Model file for the job. Use its own axes, mm. A direction names the side the tool comes from. Coordinates: 2 decimals unless noted, no trailing zeros. Order: outer loops, then holes, each group sorted by start corner. A loop starts at its lowest first (then second) coordinate and runs counter-clockwise, first axis right, second up.
from build123d import *

# Parameters (mm, degrees)
SKETCH2_W               = 180
SKETCH2_H               = 9
BOSS_EXTRUDE1_DEPTH     = 14.8
SKETCH7_W               = 180
SKETCH7_H               = 4.5
CUT_EXTRUDE1_DEPTH      = 92.319713096
SKETCH8_W               = 90
SKETCH8_H               = 4.5
BOSS_EXTRUDE2_DEPTH     = 7
SKETCH10_R              = 1.5
CUT_EXTRUDE2_DEPTH      = 8
BOSS_EXTRUDE3_DEPTH     = 14.8
CUT_EXTRUDE3_DEPTH      = 178.187961437
CUT_EXTRUDE3_DEPTH_BACK = 178.187961437
SKETCH12_R              = 2
CUT_EXTRUDE4_DEPTH      = 112.397156258
CUT_EXTRUDE4_DEPTH_BACK = 112.397156258
SKETCH13_W              = 26.348017916
SKETCH13_H              = 14.929639375
FILLET2_R               = 5
CHAMFER1_SIZE           = 20


with BuildPart() as part:
    # Sketch2 → Boss-Extrude1 (new body)
    with BuildSketch(Plane(origin=(0, 0, 0), x_dir=(0, 0, -1), z_dir=(1, 0, 0))):
        Rectangle(SKETCH2_W, SKETCH2_H)
    extrude(amount=BOSS_EXTRUDE1_DEPTH)

    # Sketch7 → Cut-Extrude1 (cut, through all)
    with BuildSketch(Plane(origin=(14.8, 0, 0), x_dir=(0, 0, -1), z_dir=(1, 0, 0))):
        with Locations((0, -2.25)):
            Rectangle(SKETCH7_W, SKETCH7_H)
    extrude(amount=-CUT_EXTRUDE1_DEPTH, mode=Mode.SUBTRACT)

    # Sketch8 → Boss-Extrude2 (add)
    with BuildSketch(Plane(origin=(14.8, 0, 0), x_dir=(0, 0, -1), z_dir=(1, 0, 0))):
        with Locations((0, 2.25)):
            Rectangle(SKETCH8_W, SKETCH8_H)
    extrude(amount=BOSS_EXTRUDE2_DEPTH)

    # Sketch10 → Cut-Extrude2 (cut)
    with BuildSketch(Plane.XZ):
        with Locations(Location((17.299494937, -22.600505063, 0), (0, 0, 270))):
            Circle(SKETCH10_R)
        with Locations(Location((17.299494937, 22.600505063, 0), (0, 0, 270))):
            Circle(SKETCH10_R)
        with BuildLine():
            Line((21.8, -20.3664278), (30.172283889, -20.3664278))
            Line((30.172283889, -20.3664278), (30.172283889, -52.03884906))
            Line((30.172283889, -52.03884906), (14.8, -52.03884906))
            Line((14.8, -52.03884906), (14.8, -45))
            add(Edge.make_bspline(
                [(14.8, -45), (14.8, -29.785835575), (21.8, -29.785835575), (21.8, -20.3664278)],
                knots=[0, 0, 0, 0, 1, 1, 1, 1], degree=3))
        make_face()
        with BuildLine():
            Line((30.172283889, 52.03884906), (14.8, 52.03884906))
            Line((14.8, 52.03884906), (14.8, 45))
            add(Edge.make_bspline(
                [(14.8, 45), (14.8, 29.785835575), (21.8, 29.785835575), (21.8, 20.3664278)],
                knots=[0, 0, 0, 0, 1, 1, 1, 1], degree=3))
            Line((21.8, 20.3664278), (30.172283889, 20.3664278))
            Line((30.172283889, 20.3664278), (30.172283889, 52.03884906))
        make_face()
    extrude(amount=-CUT_EXTRUDE2_DEPTH, mode=Mode.SUBTRACT)

    # Sketch11 → Boss-Extrude3 (add)
    with BuildSketch(Plane(origin=(14.8, 0, 0), x_dir=(0, 0, -1), z_dir=(1, 0, 0))):
        with BuildLine():
            Line((74.579, 40.3), (74.579, 4.5))
            Line((74.579, 4.5), (65.579, 4.5))
            Line((65.579, 4.5), (65.579, 46.5))
            Line((65.579, 46.5), (65.579, 61.92))
            Line((65.579, 61.92), (74.579, 61.92))
            Line((74.579, 61.92), (74.579, 52.7))
            ThreePointArc((74.579, 52.7), (68.379, 46.5), (74.579, 40.3))
        make_face()
        with BuildLine():
            Line((-74.579, 52.7), (-74.579, 61.92))
            Line((-74.579, 61.92), (-65.579, 61.92))
            Line((-65.579, 61.92), (-65.579, 46.5))
            Line((-65.579, 46.5), (-65.579, 4.5))
            Line((-65.579, 4.5), (-74.579, 4.5))
            Line((-74.579, 4.5), (-74.579, 40.3))
            ThreePointArc((-74.579, 40.3), (-68.379, 46.5), (-74.579, 52.7))
        make_face()
    extrude(amount=-BOSS_EXTRUDE3_DEPTH)

    # Sketch12 → Cut-Extrude3 (cut, two sides: drawn at the far end of the back side and taken through both)
    with BuildSketch(Plane.XY.offset(74.579).offset(-CUT_EXTRUDE3_DEPTH_BACK)):
        with Locations((7.4, 57.2)):
            Circle(SKETCH12_R)
        with Locations((7.4, 35.8)):
            Circle(SKETCH12_R)
    extrude(amount=CUT_EXTRUDE3_DEPTH + CUT_EXTRUDE3_DEPTH_BACK, mode=Mode.SUBTRACT)

    # Sketch13 → Cut-Extrude4 (cut, two sides: drawn at the far end of the back side and taken through both)
    with BuildSketch(Plane.ZY.offset(-CUT_EXTRUDE4_DEPTH_BACK)):
        with Locations((87.753008958, -2.964819688)):
            Rectangle(SKETCH13_W, SKETCH13_H)
        with Locations((-87.753008958, -2.964819688)):
            Rectangle(SKETCH13_W, SKETCH13_H)
    extrude(amount=CUT_EXTRUDE4_DEPTH + CUT_EXTRUDE4_DEPTH_BACK, mode=Mode.SUBTRACT)

    # Fillet2
    fillet2_edges = [part.edges().sort_by_distance(p)[0] for p in [
        (7.4, 0, -74.579),
        (7.4, 0, 74.579),
    ]]
    fillet(fillet2_edges, radius=FILLET2_R)

    # Chamfer1
    chamfer1_edges = [part.edges().sort_by_distance(p)[0] for p in [
        (7.4, 4.5, 65.579),
        (7.4, 4.5, -65.579),
    ]]
    chamfer(chamfer1_edges, length=CHAMFER1_SIZE)


solid = part.part
Q1. Cut at C-C, the plane y = 46.5. List the corners of the cut face in (x, z).
Established:
outline: (0, -68.38) - (14.8, -68.38) - (14.8, -65.58) - (0, -65.58) - close; (0, 65.58) - (14.8, 65.58) - (14.8, 68.38) - (0, 68.38) - close
Q2. Which spindle directions (+Z, -Z, +X, -X, +Y, -Y) get a long thin tool onto all of the face, cutting with end or side? Do faces 4 (the face through (16.725, 2.218, -23.986)), 5 (the face through (21.8, 2, 0)), 6 (the face through (14.8, 25, 67)), 7 (the face through (14.8, 25, -66)), 8 (the face through (11, 4.5, 1)). Say none if no direction does.
Established:
face 4: +Y, -Y
face 5: +Z, -Z, +X, +Y, -Y
face 6: +Z, +X, +Y, -Y
face 7: -Z, +X, +Y, -Y
face 8: +X, -X, +Y
Q3. Drop flat-ended pins along their axis: P1, Ø1.8, axis at x = 17.3, z = 22.6, coming from the -Y side; P2, Ø15, axis at y = 46.5, z = -65, coming from the +X side. Give the stop position or say it passes through.
Established:
P1: passes through
P2: stops at x = 14.8
Q4. Cut at D-D, the plane z = -62.5. List the corners of the cut face in (x, y), plus the area to 3 significant figures.
Established:
outline: (0, 0) - (14.8, 0) - (14.8, 21.42) - (0, 21.42) - close
area: 317 mm2
Q5. Mould opens along Z. For faces 1 (the face through (8.323, 55.426, 70.016)), 2 (the face through (8, 55, 74.579)), 3 (the face through (7.5, 14.36, 55.44)) say: pulls with the +Z half, pulls with the -Z half, needs draft (parallel to the pull), parting line crosses it, or undercut.
Established:
face 1: needs draft
face 2: pulls with the +Z half
face 3: undercut
Q6. Cut at B-B, the plane y = 35.8. List the corners of the cut face in (x, z).
Established:
outline: (0, -74.58) - (5.4, -74.58) - (5.4, -65.58) - (0, -65.58) - close; (0, 65.58) - (5.4, 65.58) - (5.4, 74.58) - (0, 74.58) - close; (9.4, -74.58) - (14.8, -74.58) - (14.8, -65.58) - (9.4, -65.58) - close; (9.4, 65.58) - (14.8, 65.58) - (14.8, 74.58) - (9.4, 74.58) - close
Q7. Probe line 1 (Y direction, x = 7.4, z = 68); line 2 (Z direction, x = 3, y = 40); line 3 (X direction, y = 57, z = 69). List the from-to ranges inside material, lowest first.
Established:
line 1: y = 0 to 33.8, 37.8 to 55.2, 59.2 to 61.92
line 2: z = -74.58 to -65.58, 65.58 to 74.58
line 3: x = 0 to 5.41, 9.39 to 14.8
Q8. Cut at A-A, the plane x = 7.4. Count the separate pieces of the cut face and the enclosed holes in it, plus the area to 3 significant figures.
Established:
separate pieces: 5
enclosed holes: 0
area: 1,830 mm2
